Input: part model. Units: mm. Frame: model coordinates. Give positions to 0.01 mm unless a question says otherwise; leave off trailing zeros. Order: outer loops, then holes, each group sorted by start corner. A loop starts at its lowest first (then second) coordinate and runs counter-clockwise, first axis right, second up. Notation, with made-up numbers: M -0.5,28 L 45.5,28 A30 ccw 45.5,50 Z; hole C -37,63.25 d8. An arc over 180 degrees is marked long. Use a Markdown table: item, result.
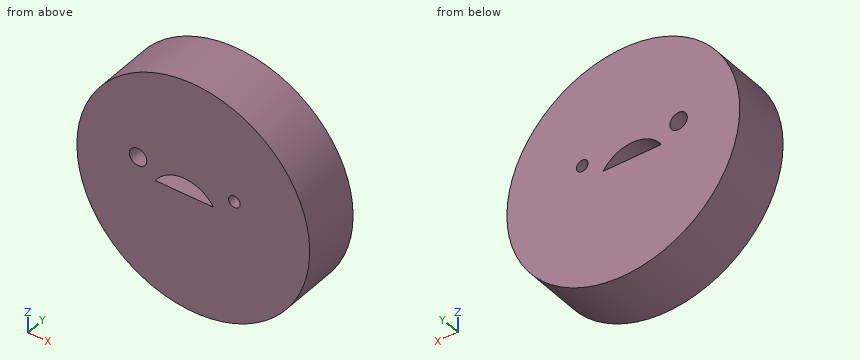
from build123d import *

# Parameters (mm, degrees)
F0_R     = 50.8
F0_R_2   = 3.81
F0_R_3   = 2.54
F1_DEPTH = 25.4


with BuildPart() as f1:
    # F0 (on Front) → F1 (new body)
    with BuildSketch(Plane.XZ):
        Circle(F0_R)
        with Locations((-24.110759, 6.902)):
            Circle(F0_R_2, mode=Mode.SUBTRACT)
        with BuildLine():
            Line((8.832272, 0), (-16.567728, 0))
            ThreePointArc((-16.567728, 0), (-3.867728, 6.902), (8.832272, 0))
        make_face(mode=Mode.SUBTRACT)
        with Locations((17.914698, 6.733317)):
            Circle(F0_R_3, mode=Mode.SUBTRACT)
    extrude(amount=F1_DEPTH)


solid = f1.part
1) Cut plane D-D on z = -38. Return loops of the section in (x, y), and give its area (3 significant figures).
Response values:
| item | result |
|---|---|
| outline | M -33.71,-25.4 L 33.71,-25.4 L 33.71,0 L -33.71,0 Z |
| area | 1,710 mm² |
2) Cut plane C-C on x = -22. Return loops of the section in (y, z).
Response values:
| item | result |
|---|---|
| outline | M -25.4,-45.79 L 0,-45.79 L 0,3.73 L -25.4,3.73 Z; M -25.4,10.07 L 0,10.07 L 0,45.79 L -25.4,45.79 Z |
3) First-contact query: pin 1 Ø1 at (x, y) = (10.5, -15.5) entering from -Z; pin 2 Ø3 at (y, z) = (-18, 40) entering from +X; pin 3 Ø1.5 at (x, y) = (-40.5, -13.5) entering from -Z. Flat tips, straight axial feed; report the tip coordinate or a pass-through.
Response values:
| item | result |
|---|---|
| pin 1 | stops at z = -49.81 |
| pin 2 | stops at x = 33.14 |
| pin 3 | stops at z = -31.63 |
4) Cut plane B-B on y = -1.75. Return loops of the section in (x, z), and give its area (3 significant figures).
Response values:
| item | result |
|---|---|
| outline | C 0,0 d101.6; hole C -24.11,6.9 d7.62; hole M -16.57,0 L 8.83,0 A15.14 ccw Z; hole C 17.91,6.73 d5.08 |
| area | 7,920 mm² |
5) Cut plane A-A on x = -2. Return loops of the section in (y, z).
Response values:
| item | result |
|---|---|
| outline | M -25.4,-50.76 L 0,-50.76 L 0,0 L -25.4,0 Z; M -25.4,6.79 L 0,6.79 L 0,50.76 L -25.4,50.76 Z |
6) Material intervals for line 1 (X direction, y = -1, z = 7); line 2 (Z direction, x = -24, y = -17); line 3 (Z direction, x = -5, y = -12.75), sorted ascending. Write a range as from..to.
Response values:
| item | result |
|---|---|
| line 1 | x = -50.32..-27.92, -20.3..15.39, 20.44..50.32 |
| line 2 | z = -44.77..3.09, 10.71..44.77 |
| line 3 | z = -50.55..0, 6.86..50.55 |
